Autodesk Fusion 360 part; units mm, degrees
sketch "Sketch1" plane through (0, 0, 0) normal (0, 0, 1) x (1, 0, 0)
  circle A0 centre (0, 0) radius 3.225
  circle A1 centre (100, 0) radius 3.225
  circle A2 centre (0, 0) radius 7.5
  circle A3 centre (100, 0) radius 7.5
  line L0 (100, 7.5) -> (0, 7.5)
  line L1 (0, -7.5) -> (100, -7.5)
  dimension "d3" = 6.45
  dimension "d4" = 6.45
  dimension "d5" = 100
  dimension "d6" = 15
  dimension "d7" = 15
extrude "Extrude1" add sketch "Sketch1" along normal blind 10 contours A2 | A3 makes body 1 at (7.4627, -0.7468, 3.3333) makes body 2 at (107.4627, -0.7468, 3.3333)
extrude "Extrude2" add sketch "Sketch1" against normal blind 5 contours A0 | A1 | A2 | A2 A3 L0 L1 | A3 bodies 1 2
equation "HoleDiam = 6.45 mm"
equation "SliderDistance = 100 mm"
equation "d3 = HoleDiam"
equation "d4 = HoleDiam"
equation "d5 = SliderDistance"
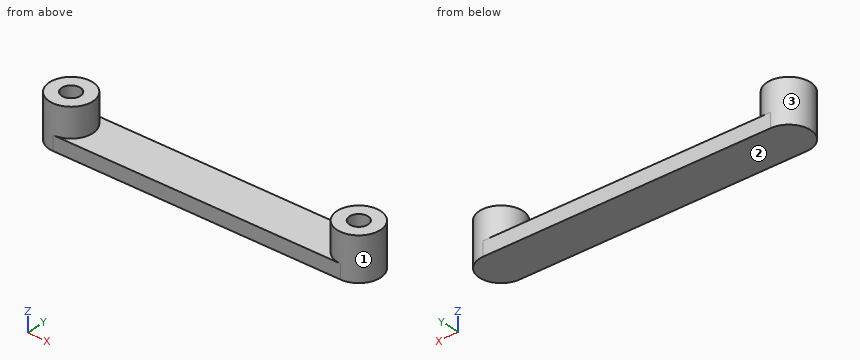
Geometry check sheet. Reference: the model listing, model coordinates, mm. Face numbers are marked on the shaded views. Coordinates: 2 decimals unless noted, no trailing zeros. Loops run counter-clockwise (first coordinate to the right, second up) from the corner with the lowest first, then second, coordinate; pieces in that order, holes last. Notation, with made-up numbers: (15, -19.75) - (69, -19.75) arc R28 cw to (69, 1.25) - close; hole circle Ø7 at (-18, -31.75). An arc over 180 degrees is marked (long way). One line per item, written item: value. Start each with the question number.
(1) Cross-section at C-C on x = 20. Enter the section's corners in (y, z).
(2) Depth check by flat-ended pin: P1, Ø6, axis at y = -3.5, z = 3.5, coming from the +X side; P2, Ø2, axis at x = 22, z = 2, coming from the +Y side; P3, Ø4.5, axis at x = 31, y = -1, coming from the +Z side; P4, Ø2, axis at y = -5, z = 7, coming from the -X side. Enter the tip coordinate at first touch or a pass-through.
(3) Cross-section at D-D on z = -4. Enter the section's corners in (x, y), plus the area to 3 significant figures.
(4) Cross-section at A-A on z = 6.5. Enter the section's corners in (x, y) (3 decimals).
(5) Cross-section at B-B on y = -5.75. Enter the section's corners in (x, z), plus the area to 3 significant figures.
(6) Mould release check, pull along X, two halves, no side actions. Record for the marked faces 1, 2 and 3: released by +X, released by -X, zero draft, split by the parting line, or undercut.
(7) Material ranges on line 1 (Y direction, x = 100, z = 3.25) (3 decimals); line 2 (X direction, y = 2.75, z = 8.75); line 3 (X direction, y = 2, z = 0.25), recorded low to high. Write a range as [from, to].
Results below:
1. outline: (-7.5, -5) - (7.5, -5) - (7.5, 0) - (-7.5, 0) - close
2. P1: stops at x = 107.48
2. P2: passes through
2. P3: stops at z = 0
2. P4: stops at x = -6.34
3. outline: (0, -7.5) - (100, -7.5) arc R7.5 ccw to (100, 7.5) - (0, 7.5) arc R7.5 ccw to start
3. area: 1,680 mm2
4. outline: circle Ø15 at (0, 0); circle Ø15 at (100, 0); hole circle Ø6.45 at (0, 0); hole circle Ø6.45 at (100, 0)
5. outline: (-4.82, -5) - (104.82, -5) - (104.82, 10) - (95.18, 10) - (95.18, 0) - (4.82, 0) - (4.82, 10) - (-4.82, 10) - close
5. area: 741 mm2
6. face 1: undercut
6. face 2: zero draft
6. face 3: undercut
7. line 1: y = [-7.5, -3.225], [3.225, 7.5]
7. line 2: x = [-6.98, -1.68], [1.68, 6.98], [93.02, 98.32], [101.68, 106.98]
7. line 3: x = [-7.23, -2.53], [2.53, 7.23], [92.77, 97.47], [102.53, 107.23]
